Source: CAD feature listing. Evaluate the final solid. Frame: model axes, mm. A direction names the side the tool comes from. Coordinates: 2 decimals unless noted, no trailing zeros. Order: outer loops, then holes, each group sorted by start corner. A loop starts at its lowest first (then second) coordinate and runs counter-clockwise, first axis right, second up.
Item 1: Contact query for flat-ended pins moving along their axis: P1, Ø4, axis at y = 0.5, z = 44, coming from the +X side; P2, Ø1, axis at x = -1, z = 40, coming from the +Y side; P3, Ø1, axis at x = -3, y = 2.5, coming from the -Z side. Output: stop coordinate, or through.
Item 2: Ray query, line 1 (X direction, y = -1, z = 26.5); line 2 (Z direction, x = 1, y = 0.5); line 3 (Z direction, x = 2.5, y = -2). Return the intervals inside material, ascending.
Item 3: Mould query, pull axis Y, two halves, no side actions, for faces 1 (the cylindrical face through (-0.54, -2.44, 29.71)), 2 (the cylindrical face through (-1.66, -0.83, 63.15)), 3 (the flat face through (0.159, 1.994, 64.26)), 4 (the flat face through (0, 0, 0)). Classes: released by +Y, released by -Y, zero draft, split by the parting line, or undercut.
Item 4: Reachability of faces 5 (the cylindrical face through (2.285, 3.584, 62.268)), 6 (the flat face through (2, -2, 60)), 7 (the flat face through (0, 0, 63)) from +Z, -Z, +X, -X, +Y, -Y: full face, straight path, thin tool, end or side. Return the list, or none.
Item 5: Section A-A on z = 16.5. Return the cut outline in (x, y).
from build123d import *

# Parameters (mm, degrees)
SKETCH1_R           = 2.5
BOSS_EXTRUDE1_DEPTH = 60
SKETCH2_R           = 4.25
BOSS_EXTRUDE2_DEPTH = 5
CUT_EXTRUDE1_DEPTH  = 2
FILLET1_R           = 0.4
CHAMFER1_SIZE       = 0.25
FILLET2_R           = 0.5


with BuildPart() as part:
    # Sketch1 → Boss-Extrude1 (new body)
    with BuildSketch(Plane.XY):
        Circle(SKETCH1_R)
    extrude(amount=BOSS_EXTRUDE1_DEPTH)

    # Sketch2 → Boss-Extrude2 (add)
    with BuildSketch(Plane.XY.offset(60)):
        Circle(SKETCH2_R)
    extrude(amount=BOSS_EXTRUDE2_DEPTH)

    # Sketch3 → Cut-Extrude1 (cut)
    with BuildSketch(Plane.XY.offset(65)):
        Polygon((2.30345988, -0.165547312), (1.295098118, 1.912081117), (-1.008361763, 2.077628429), (-2.30345988, 0.165547312), (-1.295098118, -1.912081117), (1.008361763, -2.077628429), align=None)
    extrude(amount=-CUT_EXTRUDE1_DEPTH, mode=Mode.SUBTRACT)

    # Fillet1
    fillet1_edges = [part.edges().sort_by_distance(p)[0] for p in [
        (-4.25, 0, 65),
    ]]
    fillet(fillet1_edges, radius=FILLET1_R)

    # Chamfer1
    chamfer1_edges = [part.edges().sort_by_distance(p)[0] for p in [
        (-2.5, 0, 0),
    ]]
    chamfer(chamfer1_edges, length=CHAMFER1_SIZE)

    # Fillet2
    fillet2_edges = [part.edges().sort_by_distance(p)[0] for p in [
        (1.655910822, -1.12158787, 63),
        (-0.143368178, -1.994854773, 63),
        (-1.799278999, -0.873266903, 63),
        (-1.655910822, 1.12158787, 63),
        (0.143368178, 1.994854773, 63),
        (1.799278999, 0.873266903, 63),
    ]]
    fillet(fillet2_edges, radius=FILLET2_R)


solid = part.part
Answer list:
1. P1: stops at x = 2.5
1. P2: stops at y = 2.45
1. P3: stops at z = 60
2. line 1: x = -2.29 to 2.29
2. line 2: z = 0 to 63
2. line 3: z = 60 to 65
3. face 1: split by the parting line
3. face 2: undercut
3. face 3: undercut
3. face 4: zero draft
4. face 5: +Z, -Z
4. face 6: -Z
4. face 7: +Z
5. outline: circle Ø5 at (0, 0)
